Autodesk Inventor part; units mm, degrees
ref_plane "YZ Plane" through (0, 0, 0) normal (1, 0, 0) x (0, 1, 0)
ref_plane "XZ Plane" through (0, 0, 0) normal (0, 1, 0) x (-1, 0, 0)
ref_plane "XY Plane" through (0, 0, 0) normal (0, 0, 1) x (1, 0, 0)
sketch "スケッチ1" plane through (0, 0, 0) normal (1, 0, 0) x (0, 1, 0)
  line L0 (0, 0) -> (-66, 0)
  line L1 (-66, 0) -> (-66, 302.0596)
  line L2 (-66, 302.0596) -> (0, 302.0596)
  line L3 (0, 302.0596) -> (0, 0)
  dimension "d9" = 66
extrude "押し出し1" add sketch "スケッチ1" along normal blind 20
sketch "スケッチ2" plane through (0, -66, 0) normal (0, -1, 0) x (1, 0, 0)
  point P0 (0, 0)
  point P1 (10.6073, 293.7876)
hole "穴1" at (10.6073, -66, 293.7876) direction (0, 1, 0) diameter 10 end through all
properties part number "垂直アーム(仮)" material "アルミニウム 6061"
Check sheet for the modelled part. Datum: model origin and axes. Units: mm. Round coordinates to 2 decimals unless told otherwise and drop trailing zeros. Write item = value, one per line. Start each with the question number.
Q1. Thickness scan on L1, parallel to Z at x = 7.75, y = -44; L2, parallel to Z at x = 11.75, y = -39. Record the ranges inside material, lowest first.
Q2. Release check for a two-part mould opening along Z. For faces 1 (the face through (10.387, -32.538, 298.783)), 2 (the face through (10, -33, 302.06)), 3 (the face through (10, -33, 0)), 4 (the face through (10, 0, 153)) record: pulls with the +Z half, pulls with the -Z half, needs draft (parallel to the pull), parting line crosses it, or undercut.
Q3. Depth check by flat-ended pin: P1, Ø1.5, axis at x = 15, y = -45.5, coming from the -Z side. Enter the tip coordinate at first touch or a pass-through.
Derived:
q1.L1 = 0 to 289.68, 297.89 to 302.06
q1.L2 = 0 to 288.92, 298.66 to 302.06
q2.face_1 = undercut
q2.face_2 = pulls with the +Z half
q2.face_3 = pulls with the -Z half
q2.face_4 = needs draft
q3.P1 = 0
